Can you work these out from the model? Positions are in its coordinate system, mm. Face numbers are marked on the shaded views. A direction names the side the tool comes from. Give positions to 0.01 mm unless a question says otherwise; leave off trailing zeros. Loops run counter-clockwise (first coordinate to the right, second up) from the corner with the lowest first, then second, coordinate; pieces in that order, holes last. Notation, with made-up numbers: (12.25, 65.25) -> (58.25, 65.25) arc R35 ccw to (58.25, 101.25) -> close; hole circle Ø8 at (-38.75, 89). An arc over 180 degrees is marked (long way). One line per question, with ' | ' between items.
from build123d import *

# Parameters (mm, degrees)
MAIN_FEATURES_SKETCH_W     = 25.4
MAIN_FEATURES_SKETCH_H     = 38.1
MAIN_FEATURES_SKETCH_R     = 3.2639
MAIN_FEATURES_SKETCH_W_2   = 3.5
MAIN_FEATURES_SKETCH_H_2   = 3.5
BASE_DEPTH                 = 2
SKETCH1_3_W                = 25.4
SKETCH1_3_H                = 22
SKETCH1_3_R                = 3.2639
STANDOFF_DEPTH             = 6
PEGS_START                 = 6
MAIN_FEATURES_SKETCH_4_W   = 6.5
MAIN_FEATURES_SKETCH_4_H   = 8.7
MAIN_FEATURES_SKETCH_4_H_2 = 5.3
PEGS_DEPTH                 = 2
FILLET1_R                  = 3
FILLET2_R                  = 1


with BuildPart() as part:
    # main_features_sketch → base (new body)
    with BuildSketch(Plane.XY):
        with Locations((0, 13.05)):
            Rectangle(MAIN_FEATURES_SKETCH_W, MAIN_FEATURES_SKETCH_H)
        with Locations((0, 19.4)):
            Circle(MAIN_FEATURES_SKETCH_R, mode=Mode.SUBTRACT)
        Rectangle(MAIN_FEATURES_SKETCH_W_2, MAIN_FEATURES_SKETCH_H_2, mode=Mode.SUBTRACT)
    extrude(amount=BASE_DEPTH)

    # Sketch1<3> → standoff (add)
    with BuildSketch(Plane.XY):
        with Locations((0, 21.1)):
            Rectangle(SKETCH1_3_W, SKETCH1_3_H)
        with Locations((0, 19.4)):
            Circle(SKETCH1_3_R, mode=Mode.SUBTRACT)
    extrude(amount=STANDOFF_DEPTH)

    # main_features_sketch<4> → pegs (add)
    with BuildSketch(Plane.XY.offset(PEGS_START)):
        with Locations((0, 27.75)):
            Rectangle(MAIN_FEATURES_SKETCH_4_W, MAIN_FEATURES_SKETCH_4_H)
        with Locations((0, 12.75)):
            Rectangle(MAIN_FEATURES_SKETCH_4_W, MAIN_FEATURES_SKETCH_4_H_2)
    extrude(amount=PEGS_DEPTH)

    # Fillet1
    fillet1_edges = [part.edges().sort_by_distance(p)[0] for p in [
        (12.7, -6, 1),
        (-12.7, -6, 1),
        (-12.7, 32.1, 3),
        (12.7, 32.1, 3),
        (12.7, 10.1, 4),
        (-12.7, 10.1, 4),
    ]]
    fillet(fillet1_edges, radius=FILLET1_R)

    # Fillet2
    fillet2_edges = [part.edges().sort_by_distance(p)[0] for p in [
        (3.25, 32.1, 7),
        (-3.25, 32.1, 7),
        (-3.25, 23.4, 7),
        (3.25, 23.4, 7),
        (-3.25, 15.4, 7),
        (-3.25, 10.1, 7),
        (3.25, 10.1, 7),
        (3.25, 15.4, 7),
    ]]
    fillet(fillet2_edges, radius=FILLET2_R)


solid = part.part
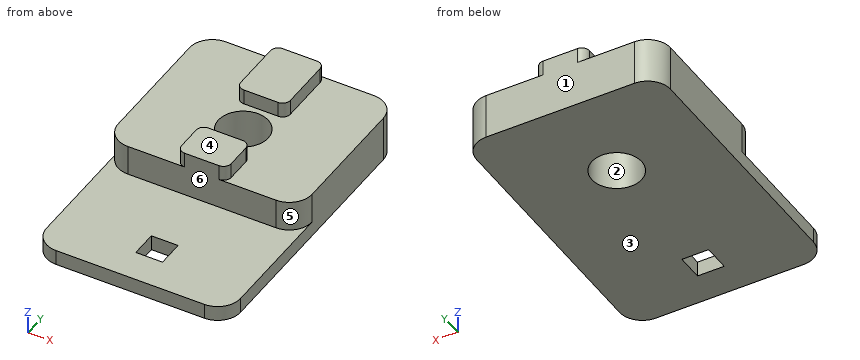
Q1. If we section it at D-D (z = 6.5): Write out the boundary of the cut face in (x, y), plus the area to 3 significant figures.
Entries:
outline: (-3.25, 11.1) arc R1 ccw to (-2.25, 10.1) -> (2.25, 10.1) arc R1 ccw to (3.25, 11.1) -> (3.25, 14.4) arc R1 ccw to (2.25, 15.4) -> (-2.25, 15.4) arc R1 ccw to (-3.25, 14.4) -> close; (-3.25, 24.4) arc R1 ccw to (-2.25, 23.4) -> (2.25, 23.4) arc R1 ccw to (3.25, 24.4) -> (3.25, 31.1) arc R1 ccw to (2.25, 32.1) -> (-2.25, 32.1) arc R1 ccw to (-3.25, 31.1) -> close | area: 89.3 mm²
Q2. For pin 1 Ø1 at (x, z) = (1, 7.5) entering from -Y; pin 2 Ø0.6 at (y, z) = (13.5, 7) entering from +X; pin 3 Ø10 at (x, y) = (5, 27) entering from +Z; pin 4 Ø1.6 at (y, z) = (28.5, 7) entering from -X, each with a flat end and sliding along its axis, tell me the tip position at first contact or that it passes through.
Entries:
pin 1: y = 10.1 | pin 2: x = 3.25 | pin 3: z = 8 | pin 4: x = -3.25
Q3. If we section it at A-A (y = 19.4): Write out the boundary of the cut face in (x, z).
Entries:
outline: (-12.7, 0) -> (-3.26, 0) -> (-3.26, 6) -> (-12.7, 6) -> close; (3.26, 0) -> (12.7, 0) -> (12.7, 6) -> (3.26, 6) -> close
Q4. On a 3-axis mill with a long thin cutter (end or side, diameter ignored), from which of +Z, -Z, +X, -X, +Y, -Y can I reach the whole of each face in a straight line? I mean the marked faces 4, 5 and 6. Say none if no direction works.
Entries:
face 4: +Z, +X, -X, +Y, -Y | face 5: +Z, +X, -Y | face 6: +Z, +X, -X, -Y
Q5. If we section it at B-B (x = 0): Write out the boundary of the cut face in (y, z), plus the area to 3 significant figures.
Entries:
outline: (-6, 0) -> (-1.75, 0) -> (-1.75, 2) -> (-6, 2) -> close; (1.75, 0) -> (16.14, 0) -> (16.14, 6) -> (15.4, 6) -> (15.4, 8) -> (10.1, 8) -> (10.1, 2) -> (1.75, 2) -> close; (22.66, 0) -> (32.1, 0) -> (32.1, 8) -> (23.4, 8) -> (23.4, 6) -> (22.66, 6) -> close | area: 146 mm²
Q6. If I drill on probe 1 along Y at (x, z) = (0, 2.1); probe 2 along X at (y, z) = (13, 3); probe 3 along Z at (x, y) = (6.25, 16.5), over which ranges is the centre line in solid material (lowest first)? Write a range as from..to.
Entries:
probe 1: 10.1..16.14, 22.66..32.1 | probe 2: -12.7..12.7 | probe 3: 0..6
Q7. If we section it at C-C (z = 3.75): Write out the boundary of the cut face in (x, y).
Entries:
outline: (-12.7, 13.1) arc R3 ccw to (-9.7, 10.1) -> (9.7, 10.1) arc R3 ccw to (12.7, 13.1) -> (12.7, 29.1) arc R3 ccw to (9.7, 32.1) -> (-9.7, 32.1) arc R3 ccw to (-12.7, 29.1) -> close; hole circle Ø6.53 at (0, 19.4)
Q8. If we mould it in two halves opening along Y, with no side actions, what happens to the marked faces 1, 2 and 3? For each: pulls with the +Y half, pulls with the -Y half, needs draft (parallel to the pull), parting line crosses it, or undercut.
Entries:
face 1: pulls with the +Y half | face 2: undercut | face 3: needs draft
